Job drawing, mm, ordinate dimensions from the low corner. One solid piece. Coordinates: 2 decimals unless noted, no trailing zeros. Order: outer loops, then holes, each group sorted by start corner. A loop starts at its lowest first (then second) coordinate and runs counter-clockwise, first axis right, second up. Notation, with made-up numbers: (-11, 65.5) - (29, 65.5) arc R12 ccw to (29, 78.5) - close; hole circle Ø4 at (84, 59.5). An arc over 180 degrees is marked (long way). Use a Markdown table: item, result. Add a question column.
1) Saw through at C-C on z = 44.5. List the corners of the cut face in (x, y), then the cut area to 3 significant figures.
2) Saw through at D-D on z = 11. List the corners of the cut face in (x, y).
3) Saw through at A-A on z = 63. List the corners of the cut face in (x, y) (1 decimal).
4) Saw through at B-B on x = 63. List the corners of the cut face in (y, z) (1 decimal).
5) Wall check: L1, parallel to X at y = 0.55, z = 63 (1 decimal); L2, parallel to Y at x = 45, z = 9; L3, parallel to Y at x = 59, z = 78.5. Give the ranges that are in metal, low to high. Write a range as [from, to].
6) Drop flat-ended pins along their axis: P1, Ø0.8, axis at x = 45.5, y = 2, coming from the -Z side; P2, Ø0.8, axis at y = 2, z = 77, coming from the -X side; P3, Ø1.5, axis at x = 37.5, y = 2, coming from the -Z side (1 decimal); P4, Ø1, axis at y = 2.5, z = 63, coming from the +X side. Give the stop position or say it passes through.
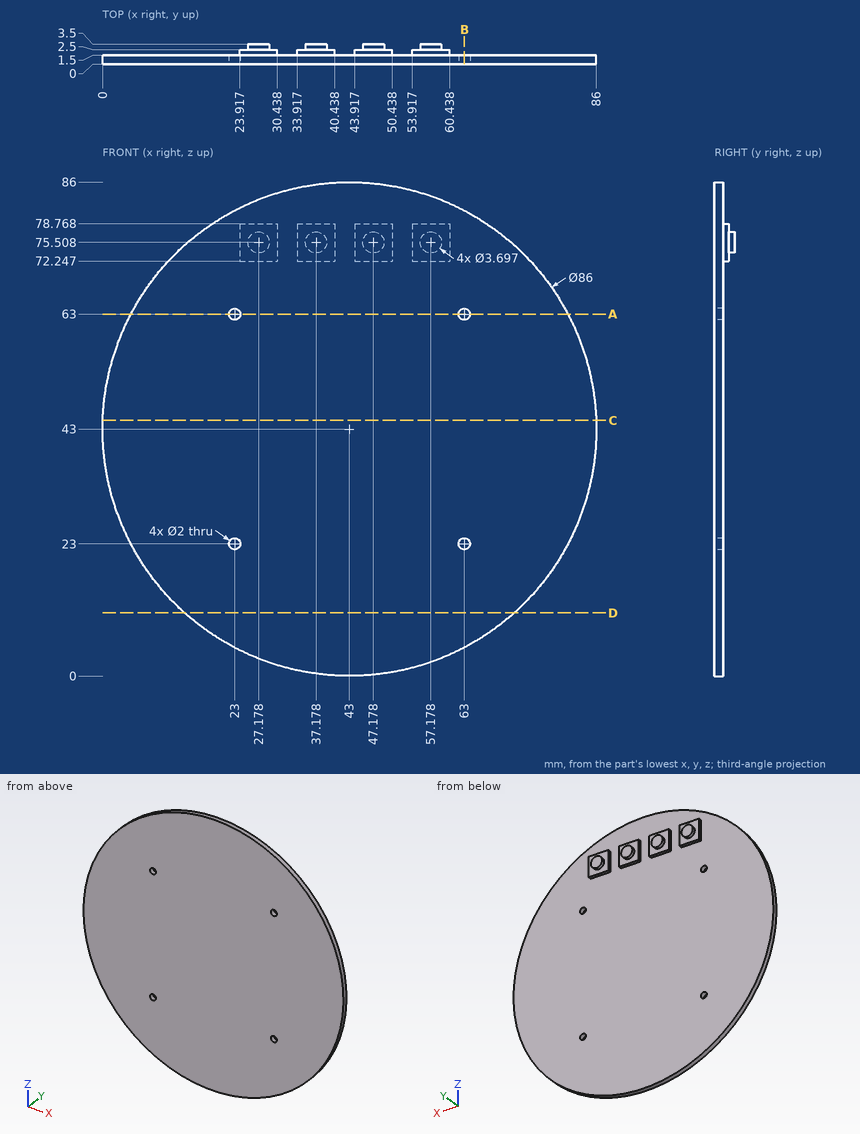
Results are:
| question | item | result |
|---|---|---|
| 1 | outline | (0.03, 0) - (85.97, 0) - (85.97, 1.5) - (0.03, 1.5) - close |
| 1 | area | 129 mm2 |
| 2 | outline | (14.28, 0) - (71.72, 0) - (71.72, 1.5) - (14.28, 1.5) - close |
| 3 | outline | (4.9, 0) - (22, 0) - (22, 1.5) - (4.9, 1.5) - close; (24, 0) - (62, 0) - (62, 1.5) - (24, 1.5) - close; (64, 0) - (81.1, 0) - (81.1, 1.5) - (64, 1.5) - close |
| 4 | outline | (0, 4.9) - (1.5, 4.9) - (1.5, 22) - (0, 22) - close; (0, 24) - (1.5, 24) - (1.5, 62) - (0, 62) - close; (0, 64) - (1.5, 64) - (1.5, 81.1) - (0, 81.1) - close |
| 5 | L1 | [4.9, 22], [24, 62], [64, 81.1] |
| 5 | L2 | [0, 1.5] |
| 5 | L3 | [0, 2.5] |
| 6 | P1 | z = 72.25 |
| 6 | P2 | x = 23.92 |
| 6 | P3 | z = 0.3 |
| 6 | P4 | through |
